```python
from build123d import *

# Parameters (mm, degrees)
F4_D     = 16
F4_DEPTH = 302.871


# Not quite as in the source:
# - a fillet or chamfer that OpenCascade refuses, or shapes differently, is made with other operations: its cross-section is extruded or revolved along the edge and cut away or added


with BuildPart() as f1:
    # F0 (on Top) → F1 (revolve)
    with BuildSketch(Plane.XY):
        with BuildLine():
            Line((0, 302.87), (-100, 302.87))
            Line((-100, 302.87), (-100, 240.87))
            ThreePointArc((-100, 240.87), (-113.9805777598, 238.2047342639), (-126, 230.5828129211))
            Line((-126, 230.5828129211), (-126, 175.1571870789))
            ThreePointArc((-126, 175.1571870789), (-113.9805777598, 167.5352657361), (-100, 164.87))
            Line((-100, 164.87), (-100, 102.87))
            Line((-100, 102.87), (0, 102.87))
            Line((0, 102.87), (0, 157.87))
            ThreePointArc((0, 157.87), (-22.5250139353, 163.9133093395), (-39, 180.4200556794))
            Line((-39, 180.4200556794), (-39, 225.3199443206))
            ThreePointArc((-39, 225.3199443206), (-22.5250139353, 241.8266906605), (0, 247.87))
            Line((0, 247.87), (0, 302.87))
        make_face()
    revolve(axis=Axis((-229.3646931648, 0, 0), (1, 0, 0)))

    # F2: chamfer of 9 on 2 edges, made by hand

    # F2_s1 → F2_t2 (revolve, cut)
    with BuildSketch(Plane.XY):
        with BuildLine():
            Line((-7.5, 247.2405983732), (0, 256.1147180479))
            Line((0, 256.1147180479), (0, 247.87))
            ThreePointArc((0, 247.87), (-3.8908074648, 247.7014802039), (-7.5, 247.2405983732))
        make_face()
    revolve(axis=Axis((0, 0, 0), (1, 0, 0)), mode=Mode.SUBTRACT)

    # F2_s3 → F2_t4 (revolve, cut)
    with BuildSketch(Plane.XY):
        with BuildLine():
            Line((0, 149.6252819521), (-7.5, 158.4994016268))
            ThreePointArc((-7.5, 158.4994016268), (-3.8908074648, 158.0385197961), (0, 157.87))
            Line((0, 157.87), (0, 149.6252819521))
        make_face()
    revolve(axis=Axis((0, 0, 0), (1, 0, 0)), mode=Mode.SUBTRACT)

    # F4 (through all, one way)
    with BuildSketch(Plane.XY):
        with Locations((-77.5457248092, 302.87)):
            Circle(F4_D / 2)
    extrude(amount=-F4_DEPTH, mode=Mode.SUBTRACT)


solid = f1.part
```
The model under review builds one solid part; all positions refer to its coordinate system, in mm. A direction names the side the tool comes from. Coordinates: 2 decimals unless noted, no trailing zeros. Order: outer loops, then holes, each group sorted by start corner. A loop starts at its lowest first (then second) coordinate and runs counter-clockwise, first axis right, second up. Notation, with made-up numbers: (26.25, -22.5) -> (61.25, -22.5) arc R24 ccw to (61.25, 2.5) -> close; hole circle Ø1 at (80, -17.5). An arc over 180 degrees is marked (long way). Answer in a Markdown table with one row per item. Add a question column.
Item 1: To check wall thickness, follow probe 1 along Z at (x, y) = (-27, 0); probe 2 along Z at (x, y) = (-59.5, 0); probe 3 along Z at (x, y) = (-33.5, 0). State the ranges of each line that lie inside material, in increasing order.
Item 2: We need section C-C on x = -29. Write out the cut boundary in (y, z), plus the area to 3 significant figures.
Item 3: Mouldability with a two-part tool opening along Z and no side actions: class faces 4 (the conical face through (-0.47, -32.56, -146.61)), 5 (the flat face through (-100, -203, -133)), 6 (the cylindrical face through (-50.7, 139.756, -268.698)), 7 (the flat face through (-100, -76, -71)) as +Z half, -Z half, draft (parallel to the pull), parting line (faces both ways), or undercut.
Item 4: We need section B-B on x = -60.5. Write out the cut boundary in (y, z).
Item 5: Clearance check with flat-ended pins moving along their axes: pin 1 (1 mm diameter, centred on x = -15.5, z = -171, fed in from -Y); pin 2 (1 mm diameter, centred on x = -46.5, z = 163.5, fed in from +Y); pin 3 (2 mm diameter, centred on x = -69, y = -88.5, fed in from +Z). State where each tip first meets the part, or that it passes through.
Item 6: We need section A-A on y = 0. Write out the cut boundary in (x, z), plus the area to 3 significant figures.
Item 7: Machinability: for faces 1 (the flat face through (0, -98, 35)), 2 (the flat face through (-39, 168, 68)), 3 (the cylindrical face through (-77.72, 294.87, -26.41)), which of the approach directions +Z, -Z, +X, -X, +Y, -Y give a long, thin tool a straight path to every point of the face, cutting with its end or side? Answer none if there is none.
Final values:
| question | item | result |
|---|---|---|
| 1 | probe 1 | z = -302.87 to -238.87, -166.87 to -102.87, 102.87 to 166.87, 238.87 to 302.87 |
| 1 | probe 2 | z = -302.87 to -102.87, 102.87 to 302.87 |
| 1 | probe 3 | z = -302.87 to -232.92, -172.82 to -102.87, 102.87 to 172.82, 232.92 to 302.87 |
| 2 | outline | circle Ø605.74 at (0, 0); circle Ø336.92 at (0, 0); hole circle Ø474.56 at (0, 0); hole circle Ø205.74 at (0, 0) |
| 2 | area | 167,000 mm2 |
| 3 | face 4 | undercut |
| 3 | face 5 | draft |
| 3 | face 6 | parting line |
| 3 | face 7 | undercut |
| 4 | outline | circle Ø605.74 at (0, 0); hole circle Ø205.74 at (0, 0) |
| 5 | pin 1 | stops at y = -250.32 |
| 5 | pin 2 | stops at y = 255.27 |
| 5 | pin 3 | stops at z = 289.96 |
| 6 | outline | (-126, -230.58) arc R38 ccw to (-100, -240.87) -> (-100, -302.87) -> (0, -302.87) -> (0, -256.11) -> (-7.5, -247.24) arc R45 cw to (-39, -225.32) -> (-39, -180.42) arc R45 cw to (-7.5, -158.5) -> (0, -149.63) -> (0, -102.87) -> (-100, -102.87) -> (-100, -164.87) arc R38 ccw to (-126, -175.16) -> close; (-126, 175.16) arc R38 ccw to (-100, 164.87) -> (-100, 102.87) -> (0, 102.87) -> (0, 149.63) -> (-7.5, 158.5) arc R45 cw to (-39, 180.42) -> (-39, 225.32) arc R45 cw to (-7.5, 247.24) -> (0, 256.11) -> (0, 302.87) -> (-100, 302.87) -> (-100, 240.87) arc R38 ccw to (-126, 230.58) -> close |
| 6 | area | 37,500 mm2 |
| 7 | face 1 | +Z, -Z, +X, +Y, -Y |
| 7 | face 2 | +X |
| 7 | face 3 | -Z, +Y |
